Could you check a few things on this model? Use its own coordinates, in mm. Face numbers are marked on the shaded views. Coordinates: 2 decimals unless noted, no trailing zeros. Order: outer loops, then holes, each group sorted by start corner. A loop starts at its lowest first (then second) coordinate and runs counter-clockwise, first axis right, second up. Notation, with made-up numbers: (27, 23.25) -> (42, 23.25) arc R12 cw to (42, 38.25) -> close; hole circle Ø3 at (-9.5, -12). An arc over 180 degrees is marked (long way). Put each result on its own line as item: value. Start each with the question number.
Q1. If we section it at B-B (z = 12.5): Please give me the cut outline in (x, y).
Q2. Please list where these lines run through material, in increasing order: line 1 along Z through (x, y) = (4.75, 0); line 2 along Y through (x, z) = (0, 8.25); line 3 along X through (y, z) = (1.5, 10.5).
Q3. If we section it at A-A (y = 0): Please give me the cut outline in (x, z), and give its area (3 significant figures).
Q4. We'd pull the mould along Y, two halves only. Please class the marked faces 1, 2 and 3: +Y half, -Y half, draft (parallel to the pull), parting line (faces both ways), or undercut.
Q5. If we section it at D-D (z = 1.5): Please give me the cut outline in (x, y), and give its area (3 significant figures).
Q6. Will these pins go through, and if not, where does the flat tip stop? pin 1 (0.5 mm diameter, centred on x = 8, y = 0, fed in from -Z); pin 2 (8 mm diameter, centred on x = 7, z = 12, fed in from +Y); pin 3 (1 mm diameter, centred on y = 6.5, z = 2, fed in from +X); pin 4 (5 mm diameter, centred on x = 0, y = 0, fed in from +Z).
Q7. If we section it at C-C (x = -7.25): Please give me the cut outline in (y, z), and give its area (3 significant figures).
Autodesk Fusion 360 part; units mm, degrees
sketch "ServoSideBase" plane through (0, 0, 0) normal (0, 0, 1) x (1, 0, 0) in component "ServoSide"
  circle A0 centre (0, 0) radius 10.4
  circle A1 centre (0, 0) radius 4.1
  dimension "d3" = 20.8
  dimension "d4" = 8.2
extrude "ExtrudeServoSideBase" add sketch "ServoSideBase" along normal blind 18 in component "ServoSide"
sketch "ServoScrews" plane through (0, 0, 0) normal (0, 0, -1) x (1, 0, 0) in component "ServoSide"
  circle A0 centre (0, 0) radius 4.1
  circle A1 centre (0, 0) radius 10.4
  line L0 (0, 10.4) -> (0, -10.4) construction
  line L1 (-10.4, 0) -> (10.4, 0) construction
  circle A2 centre (0, 7.75) radius 0.8
  circle A3 centre (-7.75, 0) radius 0.8
  circle A4 centre (0, -7.75) radius 0.8
  circle A5 centre (7.75, 0) radius 0.8
  point P0 (0, 7.75)
  dimension "d7" = 7.75
  dimension "d8" = 1.6
  dimension "d10" = 360
extrude "CutServoScrewHoles" cut sketch "ServoScrews" against normal blind 4 contours A2 | A3 | A4 | A5 in component "ServoSide"
sketch "LargeScrewHole" plane through (0, 0, 0) normal (1, 0, 0) x (0, 1, 0) in component "ServoSide"
  line L0 (0, 18) -> (0, 0) construction
  circle A0 centre (0, 13.5) radius 3.3
  point P0 (0, 18)
  dimension "d41" = 6.6
  dimension "d42" = 4.5
extrude "ExtrudeScrewHole" cut sketch "LargeScrewHole" along normal through all and the other way through all in component "ServoSide"
component "ServoSide" placed x (1, 0, 0) y (0, 1, 0) z (0, 0, 1) at (0, 0, 0)
equation "outside_diam = 20.8 mm"
equation "inside_diam = 8.2 mm"
equation "d3 = outside_diam"
equation "d4 = inside_diam"
equation "d5 = servoside_height"
equation "servoside_height = 18 mm"
equation "slop = 0.1 mm"
equation "neckside_height = 16 mm"
equation "sm_screw_diam = 3.9 mm"
equation "lg_screw_diam = 6.4 mm"
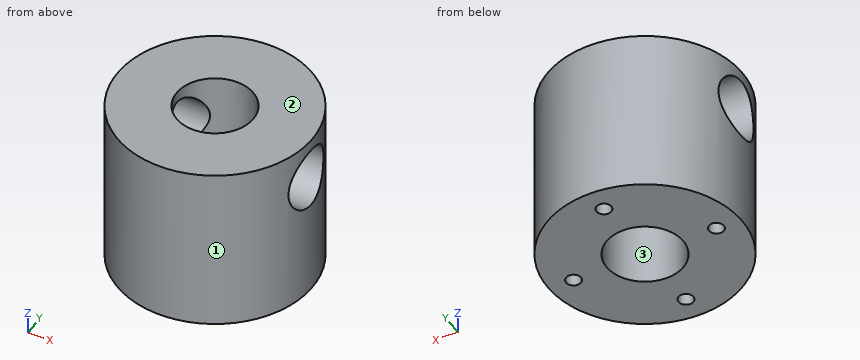
The answers:
1. outline: (-9.91, -3.14) arc R10.4 ccw to (9.91, -3.14) -> (2.63, -3.14) arc R4.1 cw to (-2.63, -3.14) -> close; (-9.91, 3.14) -> (-2.63, 3.14) arc R4.1 cw to (2.63, 3.14) -> (9.91, 3.14) arc R10.4 ccw to start
2. line 1: 0 to 10.2, 16.8 to 18
2. line 2: -10.4 to -4.1, 4.1 to 10.4
2. line 3: -10.29 to -3.82, 3.82 to 10.29
3. outline: (-10.4, 0) -> (-8.55, 0) -> (-8.55, 4) -> (-6.95, 4) -> (-6.95, 0) -> (-4.1, 0) -> (-4.1, 10.2) -> (-10.4, 10.2) -> close; (-10.4, 16.8) -> (-4.1, 16.8) -> (-4.1, 18) -> (-10.4, 18) -> close; (4.1, 0) -> (6.95, 0) -> (6.95, 4) -> (8.55, 4) -> (8.55, 0) -> (10.4, 0) -> (10.4, 10.2) -> (4.1, 10.2) -> close; (4.1, 16.8) -> (10.4, 16.8) -> (10.4, 18) -> (4.1, 18) -> close
3. area: 131 mm^2
4. face 1: parting line
4. face 2: draft
4. face 3: undercut
5. outline: circle Ø20.8 at (0, 0); hole circle Ø1.6 at (-7.75, 0); hole circle Ø8.2 at (0, 0); hole circle Ø1.6 at (0, -7.75); hole circle Ø1.6 at (0, 7.75); hole circle Ø1.6 at (7.75, 0)
5. area: 279 mm^2
6. pin 1: z = 4
6. pin 2: y = 9.96
6. pin 3: x = 8.49
6. pin 4: through
7. outline: (-7.46, 0) -> (-0.62, 0) -> (-0.62, 4) -> (0.62, 4) -> (0.62, 0) -> (7.46, 0) -> (7.46, 18) -> (-7.46, 18) -> close; hole circle Ø6.6 at (0, 13.5)
7. area: 229 mm^2
